Read the model definition and answer for the solid it produces. Units are mm, in the model's axes. A direction names the side the tool comes from. Coordinates: 2 decimals unless noted, no trailing zeros. Write each loop counter-clockwise with the first axis right and the second up, starting at its lowest first coordinate (ties: lowest second). Pieces come first, ordered by that corner, then holes. Notation, with made-up numbers: (-18, 77.25) -> (40, 77.25) arc R17 cw to (40, 110.25) -> close; hole circle Ø11 at (49, 50). An arc over 180 degrees is marked (long way). Answer as a JSON object with one key per item and string values. Group by question number.
(1) Which of the six approach directions +Z, -Z, +X, -X, +Y, -Y give full straight-line access (tool end or side, diameter ignored) to faces 1 (the face through (-1, 81, 12.7)), 2 (the face through (292.1, -1, 6))?
(2) Find section B-B (x = 164.5). Give the vertices of the cut face in (y, z).
(3) Flat-ended cylindrical pins translate along their axes: P1, Ø4, axis at x = -239, z = 1.5, coming from the -Y side; P2, Ø3, axis at y = 60, z = 8.5, coming from the +X side. Find the tip coordinate at first contact, or state that the pin passes through.
(4) Straight lines are drawn through the part: L1, parallel to Y at x = 67.5, z = 6; L2, parallel to Y at x = -83, z = 8.5; L3, parallel to X at y = -64, z = 4.5. For each, find the intervals that lie inside material, in ascending order.
(5) For a pull along Y with two mould halves and no side action, classify faces 3 (the face through (-292.1, -1, 6)), 4 (the face through (-1, 81, 0)) as +Y half, -Y half, draft (parallel to the pull), parting line (faces both ways), or undercut.
(6) Find section C-C (z = 10.5). Give the vertices of the cut face in (x, y), then the cut area to 3 significant figures.
(7) Find section A-A (y = 49). Give the vertices of the cut face in (x, z), then the cut area to 3 significant figures.
from build123d import *

# Parameters (mm, degrees)
F0_W     = 609.6
F0_H     = 177.8
F0_W_2   = 584.2
F0_H_2   = 152.4
F1_DEPTH = 12.7
F2_R     = 5.08


with BuildPart() as f1:
    # F0 (on Top) → F1 (new body)
    with BuildSketch(Plane.XY):
        Rectangle(F0_W, F0_H)
        Rectangle(F0_W_2, F0_H_2, mode=Mode.SUBTRACT)
    extrude(amount=F1_DEPTH)

    # F2
    f2_edges = [f1.edges().sort_by_distance(p)[0] for p in [
        (0, -88.9, 12.7),
        (-304.8, 0, 12.7),
        (304.8, 0, 0),
        (0, 88.9, 12.7),
        (304.8, 88.9, 6.35),
        (304.8, -88.9, 6.35),
        (-304.8, -88.9, 6.35),
        (-304.8, 88.9, 6.35),
        (304.8, 0, 12.7),
        (0, -88.9, 0),
        (0, 88.9, 0),
        (-304.8, 0, 0),
    ]]
    fillet(f2_edges, radius=F2_R)


solid = f1.part
Results below:
{
 "1": {"face 1": "+Z, +X, -X, +Y, -Y", "face 2": "+Z, -Z"},
 "2": {"outline": "(-88.9, 5.08) arc R5.08 ccw to (-83.82, 0) -> (-76.2, 0) -> (-76.2, 12.7) -> (-83.82, 12.7) arc R5.08 ccw to (-88.9, 7.62) -> close; (76.2, 0) -> (83.82, 0) arc R5.08 ccw to (88.9, 5.08) -> (88.9, 7.62) arc R5.08 ccw to (83.82, 12.7) -> (76.2, 12.7) -> close"},
 "3": {"P1": "stops at y = -88.65", "P2": "stops at x = 304.8"},
 "4": {"L1": "y = -88.9 to -76.2, 76.2 to 88.9", "L2": "y = -88.82 to -76.2, 76.2 to 88.82", "L3": "x = -304.77 to -292.1, 292.1 to 304.77"},
 "5": {"face 3": "undercut", "face 4": "draft"},
 "6": {"outline": "(-303.9, -83.82) arc R4.18 ccw to (-299.72, -88) -> (299.72, -88) arc R4.18 ccw to (303.9, -83.82) -> (303.9, 83.82) arc R4.18 ccw to (299.72, 88) -> (-299.72, 88) arc R4.18 ccw to (-303.9, 83.82) -> close; hole (-292.1, -76.2) -> (292.1, -76.2) -> (292.1, 76.2) -> (-292.1, 76.2) -> close", "area": "17,900 mm2"},
 "7": {"outline": "(-304.8, 5.08) arc R5.08 ccw to (-299.72, 0) -> (-292.1, 0) -> (-292.1, 12.7) -> (-299.72, 12.7) arc R5.08 ccw to (-304.8, 7.62) -> close; (292.1, 0) -> (299.72, 0) arc R5.08 ccw to (304.8, 5.08) -> (304.8, 7.62) arc R5.08 ccw to (299.72, 12.7) -> (292.1, 12.7) -> close", "area": "300 mm2"}
}
